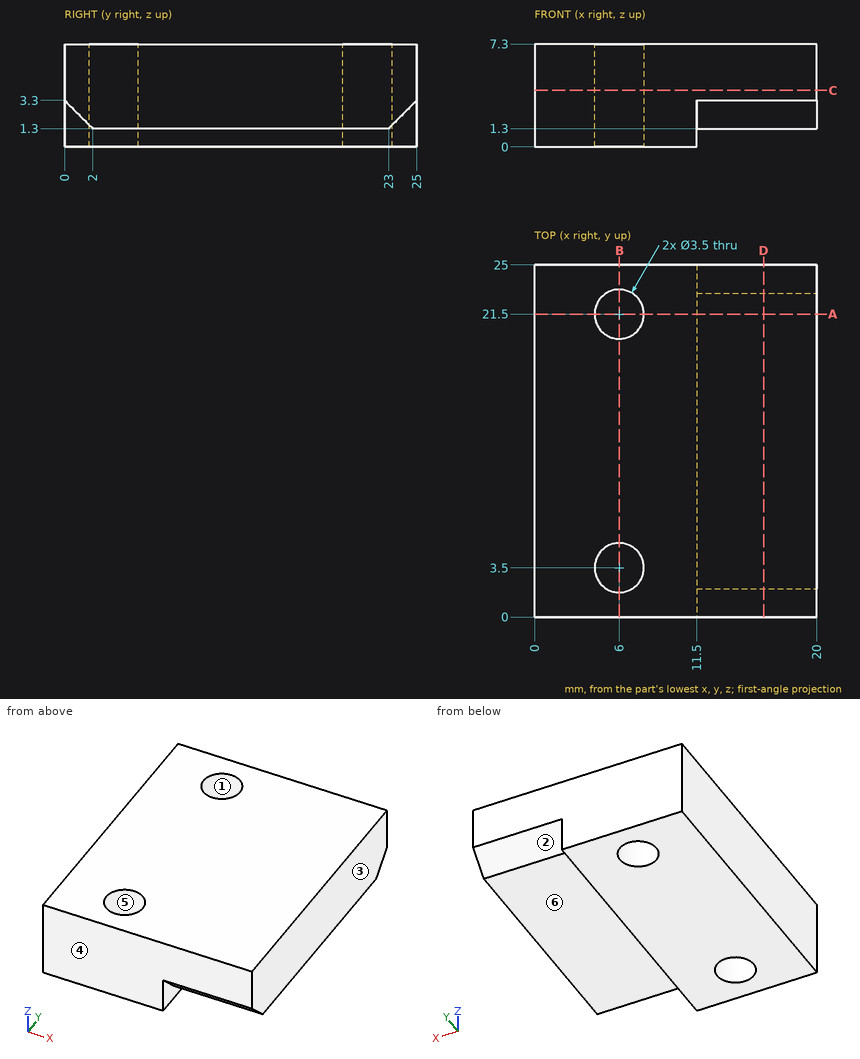
The drawing under review shows one solid part. Ordinate dimensions are in mm from its lowest x, y, z. A direction names the side the tool comes from. Round coordinates to 2 decimals unless told otherwise and drop trailing zeros. Loops run counter-clockwise (first coordinate to the right, second up) from the corner with the lowest first, then second, coordinate; pieces in that order, holes last. Notation, with made-up numbers: (36.5, 53.5) -> (61.5, 53.5) arc R25 ccw to (61.5, 90.5) -> close; hole circle Ø8 at (-32.5, 36.5). An arc over 180 degrees is marked (long way). One line per question, with ' | ' between items. Start each with the question number.
Item 1: Add section D-D, the plane x = 16.25. Write out the cut boundary in (y, z), then the cut area to 3 significant figures.
Item 2: Machinability: for the marked faces 5 and 6, which of the approach directions +Z, -Z, +X, -X, +Y, -Y give a long, thin tool a straight path to every point of the face, cutting with its end or side? Answer none if there is none.
Item 3: Add section C-C, the plane z = 4. Write out the cut boundary in (x, y).
Item 4: Add section B-B, the plane x = 6. Write out the cut boundary in (y, z).
Item 5: Draft analysis for pull direction Y (two halves, no side actions). For the marked faces 1, 2, 3 and 4, state which applies: +Y half, -Y half, draft (parallel to the pull), parting line (faces both ways), or undercut.
Item 6: Wall thickness on line 1 along Y through (x, z) = (6, 2.75); line 2 along X through (y, z) = (20.25, 3.25); line 3 along Y through (x, z) = (7, 1): over which ranges is each line inside the solid? List them lowest first. Write a range as [from, to].
Item 7: For pin 1 (2.5 mm diameter, centred on x = 15.5, y = 12, fed in from -Z), flat-tipped, find the tip position at first contact; note if it passes through.
Item 8: Add section A-A, the plane y = 21.5. Write out the cut boundary in (x, z).
Return value:
1) outline: (0, 3.3) -> (2, 1.3) -> (23, 1.3) -> (25, 3.3) -> (25, 7.3) -> (0, 7.3) -> close | area: 146 mm2
2) face 5: +Z, -Z | face 6: -Z, +X, +Y, -Y
3) outline: (0, 0) -> (20, 0) -> (20, 25) -> (0, 25) -> close; hole circle Ø3.5 at (6, 3.5); hole circle Ø3.5 at (6, 21.5)
4) outline: (0, 0) -> (1.75, 0) -> (1.75, 7.3) -> (0, 7.3) -> close; (5.25, 0) -> (19.75, 0) -> (19.75, 7.3) -> (5.25, 7.3) -> close; (23.25, 0) -> (25, 0) -> (25, 7.3) -> (23.25, 7.3) -> close
5) face 1: undercut | face 2: +Y half | face 3: draft | face 4: -Y half
6) line 1: y = [0, 1.75], [5.25, 19.75], [23.25, 25] | line 2: x = [0, 4.78], [7.22, 20] | line 3: y = [0, 2.06], [4.94, 20.06], [22.94, 25]
7) pin 1: stops at z = 1.3
8) outline: (0, 0) -> (4.25, 0) -> (4.25, 7.3) -> (0, 7.3) -> close; (7.75, 0) -> (11.5, 0) -> (11.5, 1.3) -> (20, 1.3) -> (20, 7.3) -> (7.75, 7.3) -> close
